Part model, mm, in its own coordinate system. A direction names the side the tool comes from. Give positions to 0.01 mm unless a question says otherwise; leave off trailing zeros. Write each loop counter-clockwise with the first axis right and the second up, starting at its lowest first coordinate (ties: lowest second). Pieces come first, ordered by that corner, then holes.
from build123d import *

# Parameters (mm, degrees)
SKETCH1_R           = 36.124355653
BOSS_EXTRUDE1_DEPTH = 1.5
SKETCH3_R           = 75
SKETCH3_R_2         = 43.124355653
BOSS_EXTRUDE2_DEPTH = 1.5
SKETCH4_R           = 75
BOSS_EXTRUDE3_DEPTH = 1
SKETCH5_R           = 27.5
SKETCH5_R_2         = 2.75
BOSS_EXTRUDE4_DEPTH = 20
CUT_EXTRUDE1_DEPTH  = 4


with BuildPart() as part:
    # Sketch1 → Boss-Extrude1 (new body)
    with BuildSketch(Plane(origin=(0, 0, 0), x_dir=(1, 0, 0), z_dir=(0, 1, 0))):
        with Locations(Location((0, 0, 0), (0, 0, 270))):
            Circle(SKETCH1_R)
    extrude(amount=BOSS_EXTRUDE1_DEPTH)



with BuildPart() as body_2:
    # Sketch3 → Boss-Extrude2 (new body)
    with BuildSketch(Plane(origin=(0, 0, 0), x_dir=(1, 0, 0), z_dir=(0, 1, 0))):
        with Locations(Location((0, 0, 0), (0, 0, 270))):
            Circle(SKETCH3_R)
        with Locations(Location((0, 0, 0), (0, 0, 270))):
            Circle(SKETCH3_R_2, mode=Mode.SUBTRACT)
    extrude(amount=BOSS_EXTRUDE2_DEPTH)


with BuildPart() as part_1:
    add(part.part)

    add(body_2.part)  # Boss-Extrude3 merges body 2
    # Sketch4 → Boss-Extrude3 (add)
    with BuildSketch(Plane(origin=(0, 1.5, 0), x_dir=(1, 0, 0), z_dir=(0, 1, 0))):
        with Locations(Location((0, 0, 0), (0, 0, 270))):
            Circle(SKETCH4_R)
    extrude(amount=BOSS_EXTRUDE3_DEPTH)

    # Sketch5 → Boss-Extrude4 (add)
    with BuildSketch(Plane(origin=(0, 2.5, 0), x_dir=(1, 0, 0), z_dir=(0, 1, 0))):
        with Locations(Location((0, 0, 0), (0, 0, 270))):
            Circle(SKETCH5_R)
        with Locations(Location((0, 0, 0), (0, 0, 270))):
            Circle(SKETCH5_R_2, mode=Mode.SUBTRACT)
        with BuildLine():
            Line((-1.25, 5.868347297), (-1.25, 24.968730444))
            ThreePointArc((-1.25, 24.968730444), (-14.694631307, 20.225424859), (-23.36040255, 8.904582681))
            Line((-23.36040255, 8.904582681), (-5.194858694, 3.002239689))
            ThreePointArc((-5.194858694, 3.002239689), (-3.526711514, 4.854101966), (-1.25, 5.868347297))
        make_face(mode=Mode.SUBTRACT)
        with BuildLine():
            Line((1.25, 5.868347297), (1.25, 24.968730444))
            ThreePointArc((1.25, 24.968730444), (14.694631307, 20.225424859), (23.36040255, 8.904582681))
            Line((23.36040255, 8.904582681), (5.194858694, 3.002239689))
            ThreePointArc((5.194858694, 3.002239689), (3.526711514, 4.854101966), (1.25, 5.868347297))
        make_face(mode=Mode.SUBTRACT)
        with BuildLine():
            Line((5.96740118, 0.624598398), (24.132945036, 6.52694139))
            ThreePointArc((24.132945036, 6.52694139), (23.776412907, -7.725424859), (15.687522767, -19.465395692))
            Line((15.687522767, -19.465395692), (4.46059924, -4.012861127))
            ThreePointArc((4.46059924, -4.012861127), (5.706339098, -1.854101966), (5.96740118, 0.624598398))
        make_face(mode=Mode.SUBTRACT)
        with BuildLine():
            Line((2.438056754, -5.482324258), (13.664980281, -20.934858823))
            ThreePointArc((13.664980281, -20.934858823), (0, -25), (-13.664980281, -20.934858823))
            Line((-13.664980281, -20.934858823), (-2.438056754, -5.482324258))
            ThreePointArc((-2.438056754, -5.482324258), (0, -6), (2.438056754, -5.482324258))
        make_face(mode=Mode.SUBTRACT)
        with BuildLine():
            Line((-4.46059924, -4.012861127), (-15.687522767, -19.465395692))
            ThreePointArc((-15.687522767, -19.465395692), (-23.776412907, -7.725424859), (-24.132945036, 6.52694139))
            Line((-24.132945036, 6.52694139), (-5.96740118, 0.624598398))
            ThreePointArc((-5.96740118, 0.624598398), (-5.706339098, -1.854101966), (-4.46059924, -4.012861127))
        make_face(mode=Mode.SUBTRACT)
    extrude(amount=BOSS_EXTRUDE4_DEPTH)

    # Sketch6 → Cut-Extrude1 (cut)
    with BuildSketch(Plane.XZ):
        Polygon((-4, 2.309401077), (-4, -2.309401077), (0, -4.618802154), (4, -2.309401077), (4, 2.309401077), (0, 4.618802154), align=None)
    extrude(amount=-CUT_EXTRUDE1_DEPTH, mode=Mode.SUBTRACT)


solid = part_1.part
1) Saw through at A-A (y = 18.75). Write the cut outline in (x, z).
Check result:
outline: circle Ø55 at (0, 0); hole (-24.13, -6.53) - (-5.97, -0.62) arc R6 cw to (-4.46, 4.01) - (-15.69, 19.47) arc R25 ccw to start; hole (-23.36, -8.9) arc R25 ccw to (-1.25, -24.97) - (-1.25, -5.87) arc R6 cw to (-5.19, -3) - close; hole (-13.66, 20.93) - (-2.44, 5.48) arc R6 cw to (2.44, 5.48) - (13.66, 20.93) arc R25 ccw to start; hole circle Ø5.5 at (0, 0); hole (1.25, -24.97) arc R25 ccw to (23.36, -8.9) - (5.19, -3) arc R6 cw to (1.25, -5.87) - close; hole (4.46, 4.01) arc R6 cw to (5.97, -0.62) - (24.13, -6.53) arc R25 ccw to (15.69, 19.47) - close
2) 3-axis set-ups, long thin cutter, end or side, ignore diameter. For faces 3 (the flat face through (2.2, 22.5, -2.2)), 4 (the flat face through (10.153, 12.36, 11.847)), 5 (the flat face through (-3, 4, -1)): which of +Z, -Z, +X, -X, +Y, -Y reach the whole face in a straight line?
Check result:
face 3: +Z, -Z, +X, -X, +Y
face 4: +Y
face 5: -Y
3) Mould opens along X. For faces 1 (the cylindrical face through (0, 12, 25)), 2 (the flat face through (-32, 2.5, -1)) say: +X half, -X half, draft (parallel to the pull), parting line (faces both ways), or undercut.
Check result:
face 1: undercut
face 2: draft
4) Saw through at B-B (z = -45). Write the cut outline in (x, y).
Check result:
outline: (-60, 0) - (60, 0) - (60, 2.5) - (-60, 2.5) - close
5) Saw through at C-C (x = -61). Write the cut outline in (y, z).
Check result:
outline: (0, -43.63) - (2.5, -43.63) - (2.5, 43.63) - (0, 43.63) - close
6) Saw through at D-D (z = -20). Write the cut outline in (x, y), and give its area (3 significant figures).
Check result:
outline: (-72.28, 0) - (-38.21, 0) - (-38.21, 1.5) - (-30.08, 1.5) - (-30.08, 0) - (30.08, 0) - (30.08, 1.5) - (38.21, 1.5) - (38.21, 0) - (72.28, 0) - (72.28, 2.5) - (18.87, 2.5) - (18.87, 22.5) - (15, 22.5) - (15, 2.5) - (1.25, 2.5) - (1.25, 22.5) - (-1.25, 22.5) - (-1.25, 2.5) - (-15, 2.5) - (-15, 22.5) - (-18.87, 22.5) - (-18.87, 2.5) - (-72.28, 2.5) - close
area: 542 mm2
7) Flat gauge pins, fed straight in: P1, Ø6.5, axis at x = 0, z = 0, coming from the -Y side; P2, Ø3, axis at x = 17, z = -31, coming from the +Y side; P3, Ø6, axis at y = 20, z = -22, coming from the -X side. Where does each tip first touch, or does it go through?
Check result:
P1: stops at y = 4
P2: stops at y = 2.5
P3: stops at x = -19.88
8) Drill centre lines: L1, parallel to X at y = 0.5, z = 0; L2, parallel to X at y = 15.5, z = 0; L3, parallel to Y at x = 35.5, z = -57. Where is each one in solid material? Low to high.
Check result:
L1: x = -75 to -43.12, -36.12 to -4, 4 to 36.12, 43.12 to 75
L2: x = -27.5 to -25, -6 to -2.75, 2.75 to 6, 25 to 27.5
L3: y = 0 to 2.5
